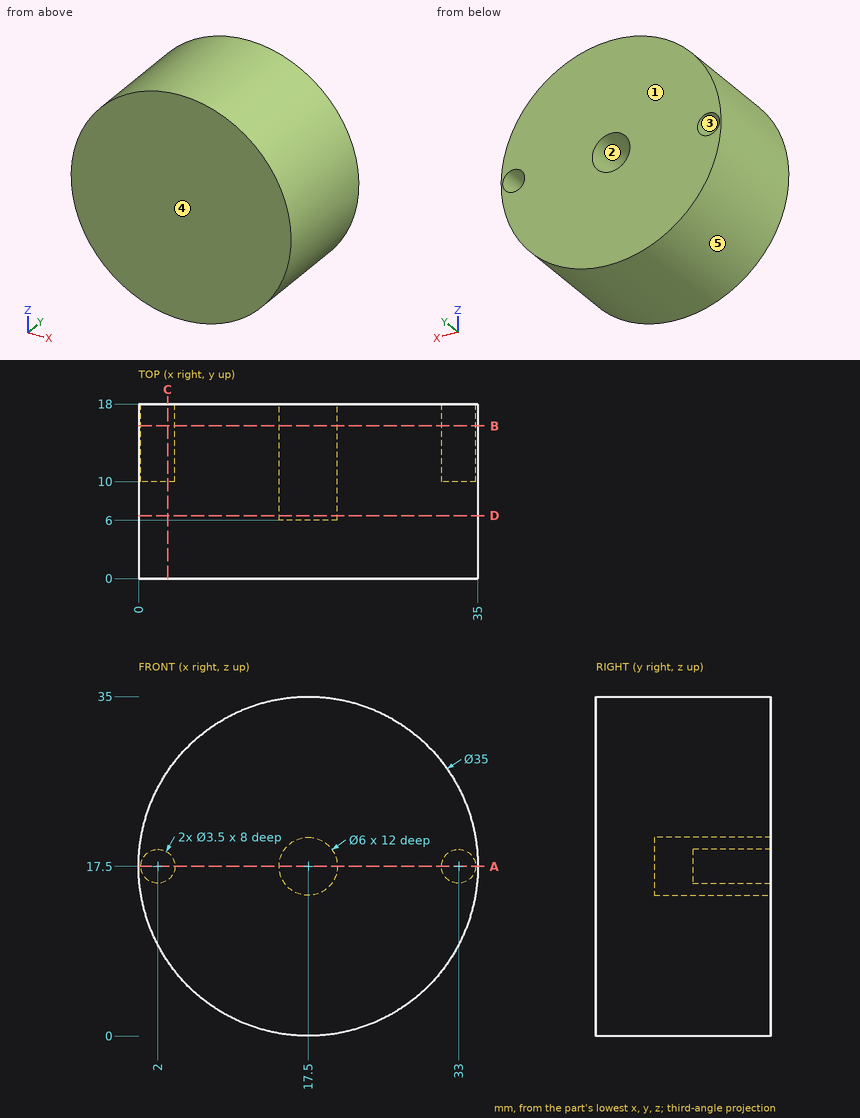
Answer from the drawing. Dimensions are ordinates in mm from the lowest x, y and z of the part. A direction names the side the tool comes from. Coordinates: 2 decimals unless noted, no trailing zeros. Write each loop counter-clockwise with the first axis right and the second up, starting at its lowest first coordinate (ties: lowest second). Pieces come first, ordered by that corner, then holes. Notation, with made-up numbers: M 75,78.25 L 109,78.25 A26 ccw 109,110.25 Z; hole C 18,87 d9. An arc over 180 degrees is marked long. Use a Markdown table: item, result.
Q1. The part is cut by section D-D, the plane y = 6.5. Write down the section's boundary in (x, z), then the cut area to 3 significant figures.
Answer block:
| item | result |
|---|---|
| outline | C 17.5,17.5 d35; hole C 17.5,17.5 d6 |
| area | 934 mm2 |
Q2. Which of the six approach directions +Z, -Z, +X, -X, +Y, -Y give full straight-line access (tool end or side, diameter ignored) to the marked faces 1 and 2?
Answer block:
| item | result |
|---|---|
| face 1 | +Z, -Z, +X, -X, +Y |
| face 2 | +Y |
Q3. The part is cut by section B-B, the plane y = 15.75. Write down the section's boundary in (x, z).
Answer block:
| item | result |
|---|---|
| outline | C 17.5,17.5 d35; hole C 2,17.5 d3.5; hole C 17.5,17.5 d6; hole C 33,17.5 d3.5 |
Q4. Each of these flat-tipped pins is pushed along its axis until it touches: pin 1 Ø2 at (y, z) = (13.5, 12) entering from +X; pin 2 Ø10 at (y, z) = (5.5, 30) entering from +X; pin 3 Ø1.8 at (x, z) = (16.5, 18.5) entering from +Y. Where does it stop, or does it pass through?
Answer block:
| item | result |
|---|---|
| pin 1 | stops at x = 34.41 |
| pin 2 | stops at x = 33.31 |
| pin 3 | stops at y = 6 |
Q5. The part is cut by section A-A, the plane z = 17.5. Write down the section's boundary in (x, y), then the cut area to 3 significant figures.
Answer block:
| item | result |
|---|---|
| outline | M 0,0 L 35,0 L 35,18 L 34.75,18 L 34.75,10 L 31.25,10 L 31.25,18 L 20.5,18 L 20.5,6 L 14.5,6 L 14.5,18 L 3.75,18 L 3.75,10 L 0.25,10 L 0.25,18 L 0,18 Z |
| area | 502 mm2 |
Q6. The part is cut by section C-C, the plane x = 3. Write down the section's boundary in (y, z).
Answer block:
| item | result |
|---|---|
| outline | M 0,7.7 L 18,7.7 L 18,16.06 L 10,16.06 L 10,18.94 L 18,18.94 L 18,27.3 L 0,27.3 Z |
Q7. Determine the mould class of the marked faces 3, 4 and 5 for opening direction Z: released by +Z, released by -Z, zero draft, split by the parting line, or undercut.
Answer block:
| item | result |
|---|---|
| face 3 | undercut |
| face 4 | zero draft |
| face 5 | split by the parting line |
Q8. Straight lines are drawn through the part: L1, parallel to X at y = 13.5, z = 17.5; L2, parallel to Z at x = 19, y = 16.5; L3, parallel to X at y = 16.5, z = 16. For each, find the intervals that lie inside material, in ascending order. Write a range as [from, to].
Answer block:
| item | result |
|---|---|
| L1 | x = [0, 0.25], [3.75, 14.5], [20.5, 31.25], [34.75, 35] |
| L2 | z = [0.06, 14.9], [20.1, 34.94] |
| L3 | x = [0.06, 1.1], [2.9, 14.9], [20.1, 32.1], [33.9, 34.94] |
